```python
from build123d import *

# Parameters (mm, degrees)
SKETCH1_R           = 1.5
BOSS_EXTRUDE1_DEPTH = 3
CUT_EXTRUDE1_DEPTH  = 10


with BuildPart() as part:
    # Sketch1 → Boss-Extrude1 (new body)
    with BuildSketch(Plane(origin=(0, 0, 0), x_dir=(1, 0, 0), z_dir=(0, 1, 0))):
        with BuildLine():
            Line((25, 5), (0, 5))
            ThreePointArc((0, 5), (-5, 0), (0, -5))
            Line((0, -5), (24.118365096, -5))
            Line((24.118365096, -5), (51.480677907, -14.959067404))
            ThreePointArc((51.480677907, -14.959067404), (57.889241728, -11.970705016), (54.90087934, -5.562141196))
            Line((54.90087934, -5.562141196), (26.710100717, 4.698463104))
            ThreePointArc((26.710100717, 4.698463104), (25.868240888, 4.924038765), (25, 5))
        make_face()
        Circle(SKETCH1_R, mode=Mode.SUBTRACT)
        with Locations((25, 0)):
            Circle(SKETCH1_R, mode=Mode.SUBTRACT)
        with Locations((53.190778624, -10.2606043)):
            Circle(SKETCH1_R, mode=Mode.SUBTRACT)
    extrude(amount=BOSS_EXTRUDE1_DEPTH)

    # Sketch2 → Cut-Extrude1 (cut)
    with BuildSketch(Plane(origin=(0, 3, 0), x_dir=(1, 0, 0), z_dir=(0, 1, 0))):
        with BuildLine():
            Line((53.619166576, -6.159813673), (57.377937059, -7.527894247))
            ThreePointArc((57.377937059, -7.527894247), (56.298907102, -6.344032156), (54.90087934, -5.562141196))
            Line((54.90087934, -5.562141196), (26.710100717, 4.698463104))
            ThreePointArc((26.710100717, 4.698463104), (29.095760221, 2.867882182), (30, 0))
            ThreePointArc((30, 0), (29.924038765, -0.868240888), (29.698463104, -1.710100717))
            Line((29.698463104, -1.710100717), (48.49231552, -8.550503583))
            Line((48.49231552, -8.550503583), (53.619166576, -6.159813673))
        make_face()
    extrude(amount=-CUT_EXTRUDE1_DEPTH, mode=Mode.SUBTRACT)


solid = part.part
```
Verification items for the finished model (mm, model axes). A direction names the side the tool comes from. Coordinates: 2 decimals unless noted, no trailing zeros. Loops run counter-clockwise (first coordinate to the right, second up) from the corner with the lowest first, then second, coordinate; pieces in that order, holes last. Notation, with made-up numbers: (59, 3) - (79, 3) arc R23 cw to (79, 22) - close; hole circle Ø10 at (-24.5, 28). An arc over 180 degrees is marked (long way). Answer as a JSON object with one key per item and string values.
(1) Scan lines: line 1 along X through (y, z) = (1.75, 0); line 2 along Z through (x, y) = (0, 1.25); line 3 along Z through (x, y) = (16, 2.05). Record each from-to range of solid material in increasing order.
Response:
{"line 1": "x = -5 to -1.5, 1.5 to 23.5, 26.5 to 30", "line 2": "z = -5 to -1.5, 1.5 to 5", "line 3": "z = -5 to 5"}
(2) Mould release check, pull along X, two halves, no side actions. Record for faces 4 (the cylindrical face through (23.5, 1.48, -0.07)), 5 (the cylindrical face through (57.05, 1.48, 13.44)), 6 (the cylindrical face through (-5, 1, 0)): pulls with the +X half, pulls with the -X half, needs draft (parallel to the pull), parting line crosses it, or undercut.
Response:
{"face 4": "undercut", "face 5": "parting line crosses it", "face 6": "pulls with the -X half"}
(3) Cross-section at B-B, the plane x = 16.5. Record the boundary of the cut face in (y, z).
Response:
{"outline": "(0, -5) - (3, -5) - (3, 5) - (0, 5) - close"}
(4) Access from +Z, -Z, +X, -X, +Y, -Y to the whole of each face (thin tool, end or side, straight path). Record for faces 1 (the flat face through (55.472, 1.521, 6.834)), 2 (the flat face through (51.02, 1.52, 7.37)), 3 (the flat face through (12, 1, 5)).
Response:
{"face 1": "-Z, +X, +Y, -Y", "face 2": "-Z, +Y, -Y", "face 3": "+Z, -X, +Y, -Y"}
(5) Go/stop test with flat-tipped pins: pin 1 Ø1.5 at (x, y) = (25.5, 1) entering from +Z; pin 2 Ø2.5 at (x, z) = (0, 0) entering from +Y; pin 3 Ø1.5 at (y, z) = (1.5, 1) entering from +X. Record where each tip stops, or that it passes through.
Response:
{"pin 1": "stops at z = 5.78", "pin 2": "passes through", "pin 3": "stops at x = 29.99"}
(6) Cross-section at A-A, the plane y = 2.05. Record the boundary of the cut face in (x, z), then the cut area to 3 significant figures.
Response:
{"outline": "(0, -5) - (25, -5) arc R5 ccw to (29.7, 1.71) - (48.49, 8.55) - (53.62, 6.16) - (57.38, 7.53) arc R5 ccw to (51.48, 14.96) - (24.12, 5) - (0, 5) arc R5 ccw to start; hole circle Ø3 at (0, 0); hole circle Ø3 at (25, 0); hole circle Ø3 at (53.19, 10.26)", "area": "487 mm²"}
(7) Cross-section at C-C, the plane z = 2.25. Record the boundary of the cut face in (x, y).
Response:
{"outline": "(-4.47, 0) - (31.18, 0) - (31.18, 3) - (-4.47, 3) - close"}
